```python
from build123d import *

# Parameters (mm, degrees)
BOSS_EXTRUDE2_DEPTH   = 167
CUT_EXTRUDE2_START    = -2
CUT_EXTRUDE2_DEPTH    = 163
SKETCH6_W             = 1
SKETCH6_H             = 1.5
SKETCH6_W_2           = 1.5
SKETCH6_H_2           = 1
BASE_SLOTS_DEPTH      = 219.342278653
SKETCH7_W             = 165
SKETCH7_H             = 138.656854249
COVER_SLOTS_DEPTH     = 1.5
COVER_SLOTS_DRAFT     = -45
USB_C_SLOTS_REACH     = 220.342
SCREEN_OVERHANG_REACH = 220.342
SKETCH9_W             = 60
SKETCH9_H             = 13.29848481


with BuildPart() as part:
    # Sketch1 → Boss-Extrude2 (new body)
    with BuildSketch(Plane(origin=(0, 0, 0), x_dir=(0, 0, -1), z_dir=(1, 0, 0))):
        Polygon((0, 0), (31.69848481, 0), (31.69848481, 2), (97.45941546, 67.76093065), (99.45941546, 67.76093065), (99.45941546, 99.45941546), align=None)
    extrude(amount=BOSS_EXTRUDE2_DEPTH)

    # Sketch5 → Cut-Extrude2 (cut)
    with BuildSketch(Plane(origin=(167, 0, 0), x_dir=(0, 0, -1), z_dir=(1, 0, 0)).offset(CUT_EXTRUDE2_START)):
        Polygon((97.45941546, 97.45941546), (2, 2), (28.870057685, 2), (97.45941546, 70.589357775), align=None)
    extrude(amount=-CUT_EXTRUDE2_DEPTH, mode=Mode.SUBTRACT)

    # Sketch6 → Base Slots (cut, through all)
    with BuildSketch(Plane(origin=(167, 0, 0), x_dir=(0, 0, -1), z_dir=(1, 0, 0))):
        with Locations((97.95941546, 68.51093065)):
            Rectangle(SKETCH6_W, SKETCH6_H)
        with Locations((30.94848481, 1.5)):
            Rectangle(SKETCH6_W_2, SKETCH6_H_2)
    extrude(amount=-BASE_SLOTS_DEPTH, mode=Mode.SUBTRACT)


with BuildPart() as cover_slots_tool:
    # Sketch7 → Cover slots (with draft: the straight prism first)
    with BuildSketch(Plane(origin=(0, 0, 0), x_dir=(1, 0, 0), z_dir=(0, 0.707106781186551, 0.7071067811865441))):
        with Locations((83.5, 70.328427125)):
            Rectangle(SKETCH7_W, SKETCH7_H)
    extrude(amount=-COVER_SLOTS_DEPTH)
    # Cover slots: the draft: its side faces are tilted about the plane it starts from
    cover_slots_sides = [cover_slots_tool.faces().sort_by_distance(p)[0] for p in [
        (1, 49.199377644, -50.260037816),
        (83.5, 0.176776695, -1.237436867),
        (166, 49.199377644, -50.260037816),
        (83.5, 98.221978593, -99.282638765),
    ]]
    draft(cover_slots_sides, Plane(origin=(0, 0, 0), x_dir=(1, 0, 0), z_dir=(0, 0.707106781186551, 0.7071067811865441)), COVER_SLOTS_DRAFT)


with BuildPart() as part_1:
    add(part.part)

    # Cover slots: cut by cover_slots_tool
    add(cover_slots_tool.part, mode=Mode.SUBTRACT)

    # Sketch8 → USB C Slots (cut, up to next)
    with BuildSketch(Plane(origin=(167, 0, 0), x_dir=(0, 0, -1), z_dir=(1, 0, 0)), mode=Mode.PRIVATE) as usb_c_slots_sk1:
        Polygon((26.162950904, 16.263455967), (62.689862838, 52.790367902), (57.74011537, 57.74011537), (21.213203436, 21.213203436), align=None)
    usb_c_slots_tool1 = extrude(usb_c_slots_sk1.sketch, amount=-USB_C_SLOTS_REACH, mode=Mode.PRIVATE) & part_1.part
    add(usb_c_slots_tool1.solids().sort_by_distance((167, 37.001786, -41.951533))[0], mode=Mode.SUBTRACT)

    # Sketch9 → Screen Overhang (cut, up to next)
    with BuildSketch(Plane(origin=(0, 0, -99.45941546), x_dir=(-1, 0, 0), z_dir=(0, 0, -1)), mode=Mode.PRIVATE) as screen_overhang_sk1:
        with Locations((-32, 92.810173055)):
            Rectangle(SKETCH9_W, SKETCH9_H)
    screen_overhang_tool1 = extrude(screen_overhang_sk1.sketch, amount=-SCREEN_OVERHANG_REACH, mode=Mode.PRIVATE) & part_1.part
    add(screen_overhang_tool1.solids().sort_by_distance((32, 92.810173, -99.459415))[0], mode=Mode.SUBTRACT)


solid = part_1.part
```
Model file for the job. Use its own axes, mm. A direction names the side the tool comes from. Give positions to 0.01 mm unless a question says otherwise; leave off trailing zeros. Loops run counter-clockwise (first coordinate to the right, second up) from the corner with the lowest first, then second, coordinate; pieces in that order, holes last. Notation, with made-up numbers: (81.5, -14) -> (140.5, -14) arc R17 ccw to (140.5, 9) -> close; hole circle Ø9 at (71.25, 82). An arc over 180 degrees is marked (long way). Use CSV: the item, a comma, the result in double quotes. Start each with the question number.
1) Slice it at D-D on y = 73. Give the cut face in (x, z), plus the area to 3 significant figures.
2) Flat gauge pins, fed straight in: pin 1 Ø1.1 at (x, z) = (68.5, -99) entering from -Y; pin 2 Ø2 at (x, y) = (66, 39) entering from -Z; pin 3 Ø5 at (x, z) = (139, -39) entering from -Y. Where does each tip first touch, or does it go through?
3) Wall check: line 1 (Y direction, x = 44, z = -25); line 2 (Z direction, x = 82.5, y = 91); line 3 (X direction, y = 53.5, z = -74). Give the ranges that are in metal, low to high.
4) Mould opens along Z. For faces 4 (the flat face through (166.014, 18.773, -23.653)), 5 (the flat face through (1.57, 48.64, -49.45)), 6 (the flat face through (101, 83, -99.459)) say: released by +Z, released by -Z, zero draft, split by the parting line, or undercut.
5) Slice it at C-C on z = -79.5. Give the cut face in (x, y), plus the area to 3 significant figures.
6) Tool access for faces 1 (the flat face through (2, 43, -55)), 2 (the flat face through (114, 99, -99)), 3 (the flat face through (166.01, 55.23, -60.25)): list every direction of +Z, -Z, +X, -X, +Y, -Y with a clear straight run to the whole face (end or side of a thin tool).
7) Slice it at A-A on x = 39. Give the cut face in (y, z).
8) Slice it at B-B on y = 88. Give the cut face in (x, z).
Computed values:
1,outline,"(0, -99.46) -> (167, -99.46) -> (167, -73) -> (166, -73) -> (165, -74.41) -> (165, -97.46) -> (2, -97.46) -> (2, -74.41) -> (1, -73) -> (0, -73) -> close"
1,area,"430 mm^2"
2,pin 1,"stops at y = 67.76"
2,pin 2,"stops at z = -69.7"
2,pin 3,"stops at y = 6.8"
3,line 1,"y = 0 to 2"
3,line 2,"z = -99.46 to -97.46"
3,line 3,"x = 0 to 2, 165 to 167"
4,face 4,"undercut"
4,face 5,"released by +Z"
4,face 6,"released by -Z"
5,outline,"(0, 49.8) -> (167, 49.8) -> (167, 79.5) -> (166, 79.5) -> (165, 78.09) -> (165, 52.63) -> (2, 52.63) -> (2, 78.09) -> (1, 79.5) -> (0, 79.5) -> close"
5,area,"578 mm^2"
6,face 1,"+Z, +Y"
6,face 2,"+Z, +X, -X, +Y"
6,face 3,"+Z, +X"
7,outline,"(0, -31.7) -> (1, -31.7) -> (1, -30.2) -> (2, -30.2) -> (2, -31.7) -> (67.76, -97.46) -> (69.26, -97.46) -> (69.26, -98.46) -> (67.76, -98.46) -> (67.76, -99.46) -> (86.16, -99.46) -> (86.16, -97.46) -> (70.59, -97.46) -> (2, -28.87) -> (2, -4.12) -> (0.71, -2.83) -> (0.71, -0.71) -> (0, 0) -> close"
8,outline,"(0, -99.46) -> (2, -99.46) -> (2, -89.41) -> (1, -88) -> (0, -88) -> close; (62, -99.46) -> (167, -99.46) -> (167, -88) -> (166, -88) -> (165, -89.41) -> (165, -97.46) -> (62, -97.46) -> close"
